from build123d import *

# Parameters (mm, degrees)
F0_W     = 44.609893
F0_H     = 51.517231
F1_DEPTH = 10.16
F2_W     = 28.780576
F2_H     = 36.55133
F3_DEPTH = 20.32
F4_W     = 16.404928
F4_H     = 24.463489
F5_DEPTH = 28.448
F6_W     = 3.02196
F6_H     = 15.253705
F7_DEPTH = 33.02


with BuildPart() as f1:
    # F0 (on Top) → F1 (new body)
    with BuildSketch(Plane.XY):
        with Locations((0.575612, 1.439029)):
            Rectangle(F0_W, F0_H)
    extrude(amount=F1_DEPTH)

    # F2 (on Top) → F3 (join)
    with BuildSketch(Plane.XY):
        with Locations((0.719515, 1.151223)):
            Rectangle(F2_W, F2_H)
    extrude(amount=F3_DEPTH)

    # F4 (on Top) → F5 (join)
    with BuildSketch(Plane.XY):
        with Locations((1.151223, 1.151224)):
            Rectangle(F4_W, F4_H)
    extrude(amount=F5_DEPTH)

    # F6 (on Top) → F7 (join)
    with BuildSketch(Plane.XY):
        with Locations((1.51098, 1.439028)):
            Rectangle(F6_W, F6_H)
    extrude(amount=F7_DEPTH)


solid = f1.part
Read the model definition and answer for the solid it produces. Units are mm, in the model's axes. A direction names the side the tool comes from. Round coordinates to 2 decimals unless told otherwise and drop trailing zeros. Write each loop counter-clockwise with the first axis right and the second up, starting at its lowest first coordinate (ties: lowest second). Pieces come first, ordered by that corner, then holes.
Q1. A tool of negligible diameter and unlimited length cuts with its end or side. For faces 1 (the face through (1, -17.124, 15)), 2 (the face through (1, 9.066, 31)), 3 (the face through (0, 1, 31)), from which of +Z, -Z, +X, -X, +Y, -Y can it reach the whole face along a straight path? Write none if from no direction.
Values:
face 1: +Z, +X, -X, -Y
face 2: +Z, +X, -X, +Y
face 3: +Z, -X, +Y, -Y
Q2. Find section D-D on y = 15. Determine the outline of the cut face in (x, z).
Values:
outline: (-21.73, 0) - (22.88, 0) - (22.88, 10.16) - (15.11, 10.16) - (15.11, 20.32) - (-13.67, 20.32) - (-13.67, 10.16) - (-21.73, 10.16) - close
Q3. Find section A-A on y = -8. Determine the outline of the cut face in (x, z), and give its area (3 significant figures).
Values:
outline: (-21.73, 0) - (22.88, 0) - (22.88, 10.16) - (15.11, 10.16) - (15.11, 20.32) - (9.35, 20.32) - (9.35, 28.45) - (-7.05, 28.45) - (-7.05, 20.32) - (-13.67, 20.32) - (-13.67, 10.16) - (-21.73, 10.16) - close
area: 879 mm2
Q4. Find section B-B on x = -12. Determine the outline of the cut face in (y, z).
Values:
outline: (-24.32, 0) - (27.2, 0) - (27.2, 10.16) - (19.43, 10.16) - (19.43, 20.32) - (-17.12, 20.32) - (-17.12, 10.16) - (-24.32, 10.16) - close
Q5. Flat-ended cylindrical pins translate along their axes: P1, Ø6.5, axis at y = -2, z = 24, coming from the -X side; P2, Ø3, axis at y = -16.5, z = 15, coming from the +X side; P3, Ø5, axis at y = 2.5, z = 30.5, coming from the +X side; P4, Ø11, axis at y = 0.5, z = 15, coming from the +X side. Find the tip coordinate at first contact, or state that the pin passes through.
Values:
P1: stops at x = -7.05
P2: stops at x = 15.11
P3: stops at x = 9.35
P4: stops at x = 22.88
Q6. Straight lines are drawn through the part: line 1 (Y direction, x = -13.5, z = 13.5); line 2 (Z direction, x = 4, y = -10); line 3 (X direction, y = -9.5, z = 22). For each, find the intervals that lie inside material, in ascending order.
Values:
line 1: y = -17.12 to 19.43
line 2: z = 0 to 28.45
line 3: x = -7.05 to 9.35
Q7. Find section C-C on z = 11.5. Determine the outline of the cut face in (x, y).
Values:
outline: (-13.67, -17.12) - (15.11, -17.12) - (15.11, 19.43) - (-13.67, 19.43) - close
